Read the model definition and answer for the solid it produces. Units are mm, in the model's axes. Coordinates: 2 decimals unless noted, no trailing zeros. Write each loop counter-clockwise with the first axis right and the second up, starting at its lowest first coordinate (ties: lowest second). Pieces come first, ordered by that corner, then holes.
(1) Straight lines are drawn through the part: line 1 along Y through (x, z) = (-153.5, 13); line 2 along X through (y, z) = (-88, 96.5); line 3 along Y through (x, z) = (-163.5, 146.5). For each, find the intervals that lie inside material, in ascending order.
(2) Determine the mould class of faces 1 (the cylindrical face through (-489.47, -465.43, 39.53)), 2 (the cylindrical face through (-512.4, -493.7, 252.9)), 3 (the flat face through (-316, -250, 0)) for opening direction Z: pulls with the +Z half, pulls with the -Z half, needs draft (parallel to the pull), parting line crosses it, or undercut.
(3) The part is cut by section A-A, the plane z = 68. Determine the outline of the cut face in (x, y) (3 decimals), and give its area (3 significant figures).
(4) Given pin 1 (10 mm diameter, centred on x = -270.5, z = 183.5, fed in from +Y); pin 2 (4 mm diameter, centred on y = -160, z = 39.5, fed in from -X); pin 3 (8 mm diameter, centred on y = -417.5, z = 175.5, fed in from -X), each flat-ended and moving along its own axis, determine where each tip first touches the part or whether it passes through.
(5) The part is cut by section B-B, the plane y = -440. Determine the outline of the cut face in (x, z).
```python
from build123d import *

# Parameters (mm, degrees)
BOSS_EXTRUDE1_DEPTH = 256.54
CUT_EXTRUDE1_REACH  = 759.98
SKETCH2_R           = 11.1125
FILLET1_R           = 12.7


with BuildPart() as part:
    # Sketch1 → Boss-Extrude1 (new body)
    with BuildSketch(Plane.XY):
        Polygon((-112.549019073, -7.182145107), (-117.475, -3.175), (-517.267555835, -494.639734243), (-512.341574908, -498.646879349), align=None)
    extrude(amount=BOSS_EXTRUDE1_DEPTH)

    # Sketch2 → Cut-Extrude1 (cut, up to next)
    with BuildSketch(Plane(origin=(-69.139884972, 56.243326117, 0), x_dir=(0, 0, 1), z_dir=(-0.77574502790219, 0.6310464734748387, 0)), mode=Mode.PRIVATE) as cut_extrude1_sk1:
        with Locations(Location((36.195, -659.334181394, 0), (0, 0, 270))):
            Circle(SKETCH2_R)
    cut_extrude1_tool1 = extrude(cut_extrude1_sk1.sketch, amount=-CUT_EXTRUDE1_REACH, mode=Mode.PRIVATE) & part.part
    # Sketch2 → Cut-Extrude1 (cut, up to next)
    with BuildSketch(Plane(origin=(-69.139884972, 56.243326117, 0), x_dir=(0, 0, 1), z_dir=(-0.77574502790219, 0.6310464734748387, 0)), mode=Mode.PRIVATE) as cut_extrude1_sk2:
        with Locations(Location((213.995, -659.334181394, 0), (0, 0, 270))):
            Circle(SKETCH2_R)
    cut_extrude1_tool2 = extrude(cut_extrude1_sk2.sketch, amount=-CUT_EXTRUDE1_REACH, mode=Mode.PRIVATE) & part.part
    add(cut_extrude1_tool1.solids().sort_by_distance((-485.210395, -455.231887, 36.195))[0], mode=Mode.SUBTRACT)
    add(cut_extrude1_tool2.solids().sort_by_distance((-485.210395, -455.231887, 213.995))[0], mode=Mode.SUBTRACT)

    # Fillet1
    fillet1_edges = [part.edges().sort_by_distance(p)[0] for p in [
        (-514.804565371, -496.643306796, 256.54),
    ]]
    fillet(fillet1_edges, radius=FILLET1_R)


solid = part.part
```
Computed:
1. line 1: y = -57.52 to -47.46
1. line 2: x = -186.48 to -178.29
1. line 3: y = -69.82 to -59.75
2. face 1: undercut
2. face 2: pulls with the +Z half
2. face 3: pulls with the -Z half
3. outline: (-517.268, -494.64) - (-512.342, -498.647) - (-112.549, -7.182) - (-117.475, -3.175) - close
3. area: 4,020 mm2
4. pin 1: stops at y = -185.14
4. pin 2: stops at x = -246.67
4. pin 3: stops at x = -457.77
5. outline: (-472.82, 0) - (-464.63, 0) - (-464.63, 256.54) - (-472.82, 256.54) - close
